Read the model definition and answer for the solid it produces. Units are mm, in the model's axes. A direction names the side the tool comes from. Coordinates: 2 decimals unless noted, no trailing zeros. Loops run counter-clockwise (first coordinate to the right, second up) from the corner with the lowest first, then second, coordinate; pieces in that order, holes last. Notation, with made-up numbers: (9, 12.25) -> (48, 12.25) arc R30 cw to (48, 42.25) -> close; hole circle Ø7 at (55.25, 65.25). An arc over 180 degrees is marked (long way). Answer in a Markdown table with one row per item.
Autodesk Inventor part; units mm, degrees
ref_plane "YZ Plane" through (0, 0, 0) normal (1, 0, 0) x (0, 1, 0)
ref_plane "XZ Plane" through (0, 0, 0) normal (0, 1, 0) x (-1, 0, 0)
ref_plane "XY Plane" through (0, 0, 0) normal (0, 0, 1) x (1, 0, 0)
sketch "Sketch1" plane through (0, 0, 0) normal (0, 0, 1) x (1, 0, 0)
  line L0 (0, 0) -> (25, 0)
  line L1 (25, 0) -> (25, 25)
  line L2 (25, 25) -> (0, 25)
  line L3 (0, 25) -> (0, 0)
  dimension "d0" = 25
extrude "Extrusion1" add sketch "Sketch1" along normal blind 5
sketch "Sketch2" plane through (0, 0, 0) normal (0, -1, 0) x (1, 0, 0)
  line L0 (0, 0) -> (25, 0)
  line L1 (25, 0) -> (25, 5)
  line L2 (0, 5) -> (25, 5)
  line L3 (0, 0) -> (0, 5)
  line L4 (0, 0) -> (25, 0)
  line L5 (25, 0) -> (25, 25)
  line L6 (25, 25) -> (0, 25)
  line L7 (0, 25) -> (0, 0)
extrude "Extrusion2" add sketch "Sketch2" against normal blind 5 contours L7 L6 L5 L2
sketch "Sketch3" plane through (0, 0, 0) normal (-1, 0, 0) x (0, 0, 1)
  line L0 (5, 25) -> (25, 25)
  line L1 (25, 25) -> (25, 5)
  line L2 (25, 5) -> (5, 5)
  line L3 (5, 5) -> (5, 25)
extrude "Extrusion3" add sketch "Sketch3" against normal blind 5
fillet "Fillet2" radius 10 6 edges at (5, 5, 15) (5, 15, 5) (15, 5, 5) (2.5, 25, 25) (25, 2.5, 25) (25, 25, 2.5)
sketch "Sketch6" plane through (0, 5, 0) normal (0, 1, 0) x (1, 0, 0)
  arc A0 (15, -25) -> (25, -15) centre (15, -15) ccw
  circle A1 centre (15, -15) radius 1.55
  point P0 (0, 0)
  dimension "d20" = 3.1
extrude "Extrusion6" cut sketch "Sketch6" along normal through all both and the other way through all
sketch "Sketch7" plane through (0, 5, 0) normal (0, 1, 0) x (1, 0, 0)
  line L0 (15, -25) -> (15, -16.55)
  arc A0 (15, -25) -> (25, -15) centre (15, -15) ccw
  line L1 (15, -18.2332) -> (12.2, -16.6166)
  line L2 (12.2, -16.6166) -> (12.2, -13.3834)
  line L3 (12.2, -13.3834) -> (15, -11.7668)
  line L4 (15, -11.7668) -> (17.8, -13.3834)
  line L5 (17.8, -13.3834) -> (17.8, -16.6166)
  line L6 (17.8, -16.6166) -> (15, -18.2332)
  point P0 (0, 0)
  dimension "d24" = 5.6
extrude "Extrusion7" cut sketch "Sketch7" along normal mid plane 5
pattern_circular "Circular Pattern2" count 3 over 360 about axis through (0, 0, 0) along (0.5774, 0.5774, 0.5774) of "Extrusion7", "Extrusion6"
properties part number "corner tab"
1. A cutting plane is placed at C-C on z = 21. Give the vertices of the cut face in (x, y), and give its area (3 significant figures).
A:
| item | result |
|---|---|
| outline | (0, 0) -> (23, 0) -> (23, 5) -> (15, 5) arc R10 cw to (5, 15) -> (5, 23) -> (0, 23) -> close |
| area | 226 mm2 |
2. A cutting plane is placed at A-A on x = 3.5. Give the vertices of the cut face in (y, z).
A:
| item | result |
|---|---|
| outline | (0, 0) -> (25, 0) -> (25, 15) arc R10 ccw to (15, 25) -> (0, 25) -> close; hole (11.77, 15) -> (13.38, 12.2) -> (16.62, 12.2) -> (18.23, 15) -> (16.62, 17.8) -> (13.38, 17.8) -> close |
3. Given pin 1 Ø3 at (y, z) = (21, 17.5) entering from +X; pin 2 Ø4.5 at (x, y) = (15.5, 15) entering from +Z; pin 3 Ø6 at (y, z) = (15.5, 15) entering from +X, each flat-ended and moving along its own axis, determine where each tip first touches the part or whether it passes through.
A:
| item | result |
|---|---|
| pin 1 | stops at x = 5 |
| pin 2 | stops at z = 2.5 |
| pin 3 | stops at x = 5.46 |
4. A cutting plane is placed at D-D on x = 17. Give the vertices of the cut face in (y, z), and give its area (3 significant figures).
A:
| item | result |
|---|---|
| outline | (0, 0) -> (24.8, 0) -> (24.8, 5) -> (17.14, 5) -> (17.14, 2.5) -> (12.86, 2.5) -> (12.86, 5.23) arc R10 cw to (5.22, 12.92) -> (2.5, 12.92) -> (2.5, 17.08) -> (5, 17.08) -> (5, 24.8) -> (0, 24.8) -> close |
| area | 223 mm2 |
5. The mould has two halves that part along Y. Classify faces 1 (the cylindrical face through (22.15, 21.99, 2.54)), 2 (the flat face through (16.4, 13.7, 2.5)), 3 (the flat face through (20, 20, 5)): pulls with the +Y half, pulls with the -Y half, needs draft (parallel to the pull), parting line crosses it, or undercut.
A:
| item | result |
|---|---|
| face 1 | pulls with the +Y half |
| face 2 | undercut |
| face 3 | needs draft |
6. A tool of negligible diameter and unlimited length cuts with its end or side. For faces 4 (the flat face through (2.5, 16.4, 13.7)), 5 (the flat face through (15, 17.8, 4)), 6 (the flat face through (12, 13, 0)), 7 (the flat face through (13.62, 3.93, 17.436)), 8 (the cylindrical face through (20.07, 7.85, 8.01)), from which of +Z, -Z, +X, -X, +Y, -Y can it reach the whole face along a straight path? Write none if from no direction.
A:
| item | result |
|---|---|
| face 4 | +X |
| face 5 | +Z |
| face 6 | -Z, +X, -X, +Y, -Y |
| face 7 | +Y |
| face 8 | +Z, +X, +Y |
7. Find the intervals of material crossed by probe 1 along Z at (x, y) = (0.7, 15), in increasing order.
A:
| item | result |
|---|---|
| probe 1 | z = 0 to 13.45, 16.55 to 25 |
8. A cutting plane is placed at B-B on y = 23.25. Give the vertices of the cut face in (x, z).
A:
| item | result |
|---|---|
| outline | (0, 0) -> (20.65, 0) -> (20.65, 5) -> (15, 5) arc R10 cw to (5, 15) -> (5, 20.65) -> (0, 20.65) -> close |
